Here's the drawing with two shaded views (mm, measured from the low corner). I have some questions. A direction names the side the tool comes from. Round coordinates to 2 decimals unless told otherwise and drop trailing zeros. Loops run counter-clockwise (first coordinate to the right, second up) from the corner with the lowest first, then second, coordinate; pieces in that order, holes last. Notation, with made-up numbers: (46, -14.5) -> (68, -14.5) arc R13 ccw to (68, -3.5) -> close; hole circle Ø4 at (-15, 47). An arc over 180 degrees is marked (long way). Write each question's results on one line, items separated by ' | '. Start each with the question number.
1) Imagine slicing it at A-A, the plane y = 36.5. List the corners of the cut face in (x, z) for me.
2) Imagine slicing it at B-B, the plane x = 136. List the corners of the cut face in (y, z) for me, plus the area to 3 significant figures.
3) If I drill on probe 1 along Z at (x, y) = (437, 42.5); probe 2 along Y at (x, z) = (351, 85.5), over which ranges is the centre line in solid material (lowest first)?
4) We'd pull the mould along Z, two halves only. Please class the marked faces 3, 4 and 5: pulls with the +Z half, pulls with the -Z half, needs draft (parallel to the pull), parting line crosses it, or undercut.
5) Imagine slicing it at C-C, the plane z = 78. List the corners of the cut face in (x, y) for me, plus the area to 3 significant figures.
6) Which directions (+Z, -Z, +X, -X, +Y, -Y) give clear straight access to the entire face, cutting with the end or side of a thin tool? Please do the marked faces 1 and 2.
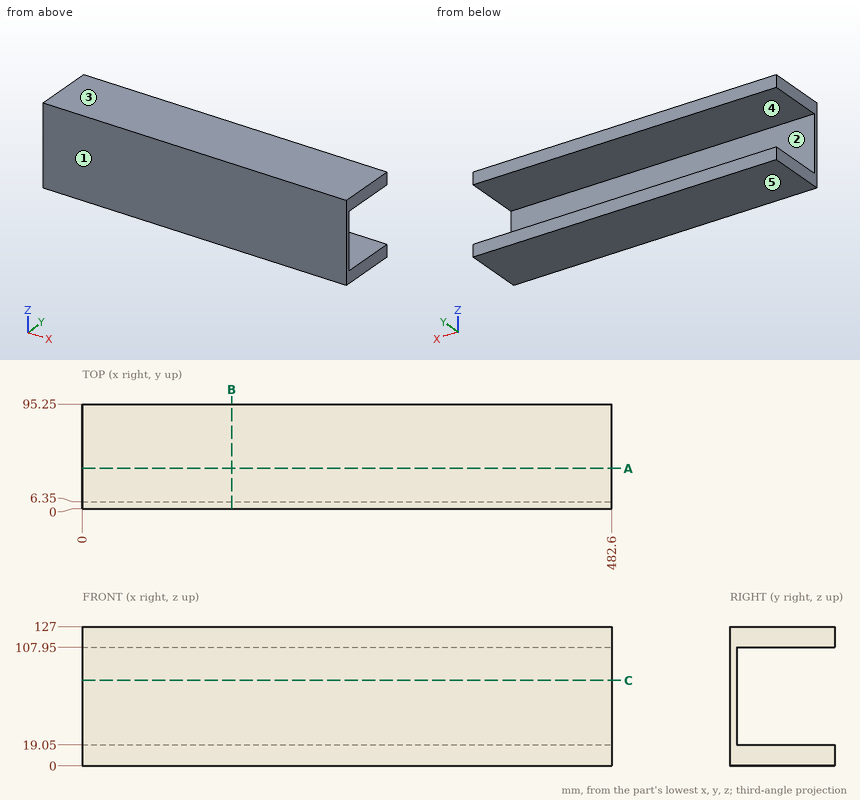
Checked values:
1) outline: (0, 0) -> (482.6, 0) -> (482.6, 19.05) -> (0, 19.05) -> close; (0, 107.95) -> (482.6, 107.95) -> (482.6, 127) -> (0, 127) -> close
2) outline: (0, 0) -> (95.25, 0) -> (95.25, 19.05) -> (6.35, 19.05) -> (6.35, 107.95) -> (95.25, 107.95) -> (95.25, 127) -> (0, 127) -> close | area: 4,190 mm^2
3) probe 1: 0 to 19.05, 107.95 to 127 | probe 2: 0 to 6.35
4) face 3: pulls with the +Z half | face 4: undercut | face 5: pulls with the -Z half
5) outline: (0, 0) -> (482.6, 0) -> (482.6, 6.35) -> (0, 6.35) -> close | area: 3,060 mm^2
6) face 1: +Z, -Z, +X, -X, -Y | face 2: +X, -X, +Y
